Check sheet for the drawn part. Datum: minimum x, y, z corner. Units: mm. Round coordinates to 2 decimals unless told otherwise and drop trailing zeros. Write each loop counter-clockwise with the first axis right and the second up, starting at its lowest first coordinate (ties: lowest second). Pieces come first, ordered by that corner, then holes.
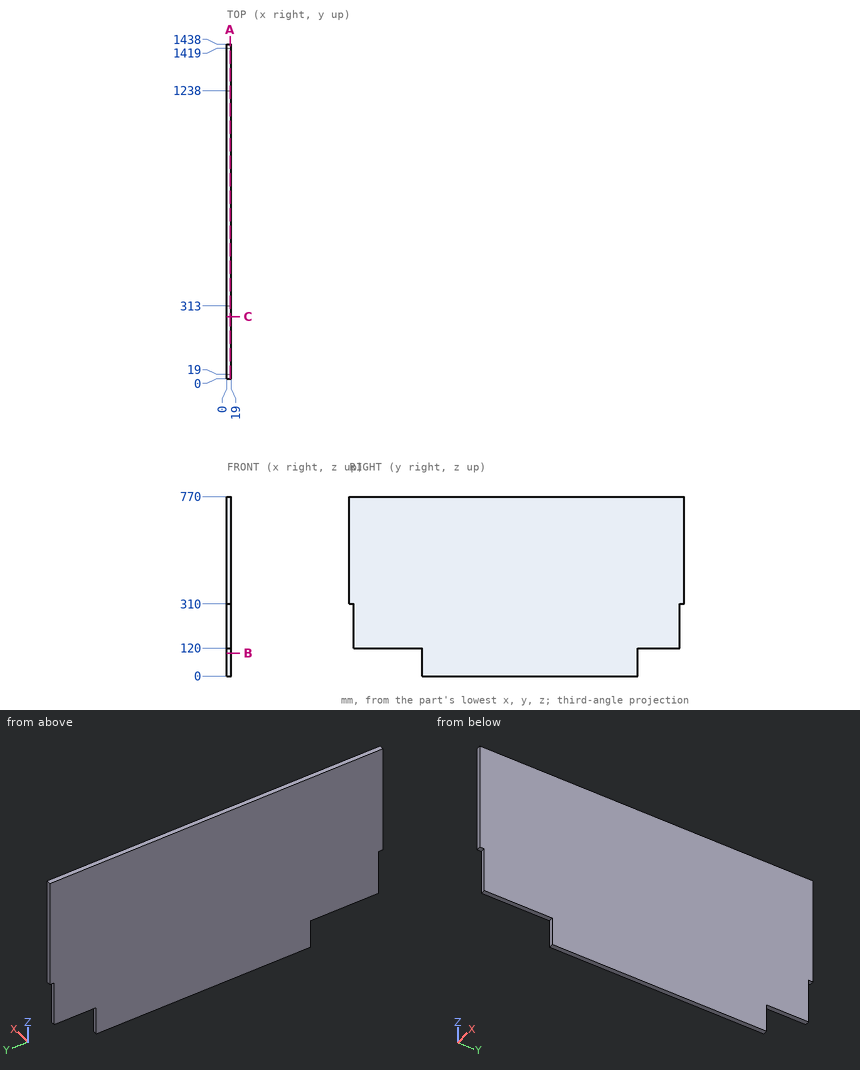
Q1. Material ranges on line 1 along Y through (x, z) = (10.5, 90.5); line 2 along Y through (x, z) = (3.75, 208); line 3 along Z through (x, y) = (9.25, 1286), recorded low to high.
Recorded:
line 1: y = 313 to 1238
line 2: y = 19 to 1419
line 3: z = 120 to 770
Q2. Sectioned sample at A-A (x = 13.5). Enter the section's corners in (y, z), plus the area to 3 significant figures.
Recorded:
outline: (0, 310) - (19, 310) - (19, 120) - (313, 120) - (313, 0) - (1238, 0) - (1238, 120) - (1419, 120) - (1419, 310) - (1438, 310) - (1438, 770) - (0, 770) - close
area: 1,040,000 mm2
Q3. Depth check by flat-ended pin: P1, Ø9.5, axis at x = 9.5, z = 61, coming from the +Y side; P2, Ø5, axis at x = 15.5, y = 693, coming from the -Z side; P3, Ø5.5, axis at x = 14, z = 44.5, coming from the -Y side; P4, Ø9.5, axis at x = 8, y = 13, coming from the -Z side. Enter the tip coordinate at first touch or a pass-through.
Recorded:
P1: stops at y = 1238
P2: stops at z = 0
P3: stops at y = 313
P4: stops at z = 310
Q4. Sectioned sample at B-B (z = 98). Enter the section's corners in (x, y), plus the area to 3 significant figures.
Recorded:
outline: (0, 313) - (19, 313) - (19, 1238) - (0, 1238) - close
area: 17,600 mm2
Q5. Sectioned sample at C-C (y = 267). Enter the section's corners in (x, z).
Recorded:
outline: (0, 120) - (19, 120) - (19, 770) - (0, 770) - close
